Check sheet for the modelled part. Datum: model origin and axes. Units: mm. Coordinates: 2 decimals unless noted, no trailing zeros. Loops run counter-clockwise (first coordinate to the right, second up) from the corner with the lowest first, then second, coordinate; pieces in that order, holes last. Notation, with made-up numbers: (35, 60.25) -> (60, 60.25) arc R23 ccw to (60, 86.25) -> close; hole circle Ø9 at (82, 70.5). An arc over 180 degrees is marked (long way). Use CSV: the item, a comma, the result in double quotes. Start each with the question number.
1. Thickness scan on L1, parallel to Z at x = -46, y = -48.5; L2, parallel to X at y = -71, z = 32; L3, parallel to X at y = -39.5, z = 46. Record the ranges inside material, lowest first.
2. Sectioned sample at A-A, the plane z = 20.5. Record the cut outline in (x, y).
3. Sectioned sample at B-B, the plane z = 47.5. Record the cut outline in (x, y).
4. Gauge pin test, flat ends, axial feed: pin 1 (3 mm diameter, centred on y = -36.5, z = 37, fed in from +X); pin 2 (1.5 mm diameter, centred on x = -53, y = -67, fed in from +Z); pin 3 (5 mm diameter, centred on x = -8.5, y = -15.5, fed in from +Z). Record the tip position at first contact, or that the pin passes through.
```python
from build123d import *

# Parameters (mm, degrees)
F1_DEPTH = 50.8
F2_R     = 17.78
F3_R     = 17.78


# Not quite as in the source:
# - a feature names something its author has since deleted; it is built from what else it names


with BuildPart() as f1:
    # F0 (on Top) → F1 (new body)
    with BuildSketch(Plane.XY):
        with BuildLine():
            Line((3.2321710605, 7.2439061478), (-50.5689829588, 7.2439061478))
            Line((-50.5689829588, 7.2439061478), (-76.5684420406, -104.0992669462))
            ThreePointArc((-76.5684420406, -104.0992669462), (-30.6491711683, -72.8314970086), (-4.5715821907, -23.7783398479))
            Line((-4.5715821907, -23.7783398479), (3.2321710605, 7.2439061478))
        make_face()
    extrude(amount=F1_DEPTH)

    # F2
    f2_edges = [f1.edges().sort_by_distance(p)[0] for p in [
        (-0.669706, -8.267217, 50.8),
        (-63.568712, -48.42768, 50.8),
    ]]
    fillet(f2_edges, radius=F2_R)

    # F3
    f3_edges = [f1.edges().sort_by_distance(p)[0] for p in [
        (-0.669706, -8.267217, 0),
        (-63.568712, -48.42768, 0),
    ]]
    fillet(f3_edges, radius=F3_R)


solid = f1.part
```
Completed:
1,L1,"0.01 to 50.79"
1,L2,"-68.84 to -29.04"
1,L3,"-55.7 to -15.86"
2,outline,"(-76.57, -104.1) arc R115.82 ccw to (-4.57, -23.78) -> (3.23, 7.24) -> (-50.57, 7.24) -> close"
3,outline,"(-65.88, -91.12) arc R108.36 ccw to (-11.81, -21.96) -> (-4.46, 7.24) -> (-42.91, 7.24) -> close"
4,pin 1,"x = -8.4"
4,pin 2,"z = 50.62"
4,pin 3,"z = 48.08"
